The figure shows three views and two pictorial views of one solid part (mm, origin at its lowest corner). Answer the questions. A direction names the side the tool comes from. Coordinates: 2 decimals unless noted, no trailing zeros. Loops run counter-clockwise (first coordinate to the right, second up) from the corner with the lowest first, then second, coordinate; pieces in that order, holes last. Notation, with made-up numbers: M 65,-15 L 87,-15 A12 cw 87,-2 Z; hole C 70,-26 d5. An arc over 180 degrees is marked long. One line per item, written item: value. Start each with the question number.
1. Consider probe 1 along Y at (x, z) = (93.5, 25.5); probe 2 along Y at (x, z) = (13, 10.5); probe 3 along X at (y, z) = (47.5, 30). Determine where each line is inside the solid, lowest interval first.
2. For the marked faces 1, 2 and 3, determine the directions among +Z, -Z, +X, -X, +Y, -Y from which every point of the face is accessible in a straight line to the end or side of a thin tool.
3. Flat-ended cylindrical pins translate along their axes: pin 1 (16.5 mm diameter, centred on y = 45.5, z = 19.5, fed in from +X); pin 2 (6 mm diameter, centred on x = 78.5, z = 16, fed in from -Y); pin 3 (8 mm diameter, centred on y = 11, z = 49.5, fed in from -X) (3 decimals); pin 4 (3 mm diameter, centred on y = 31.5, z = 32.5, fed in from -X). Find the tip coordinate at first contact, or state that the pin passes through.
4. The part is cut by section A-A (y = 26.5). Write down the section's boundary in (x, z).
5. The part is cut by section B-B (x = 49.5). Write down the section's boundary in (y, z).
6. The part is cut by section C-C (y = 12.5). Write down the section's boundary in (x, z), then the cut area to 3 significant figures.
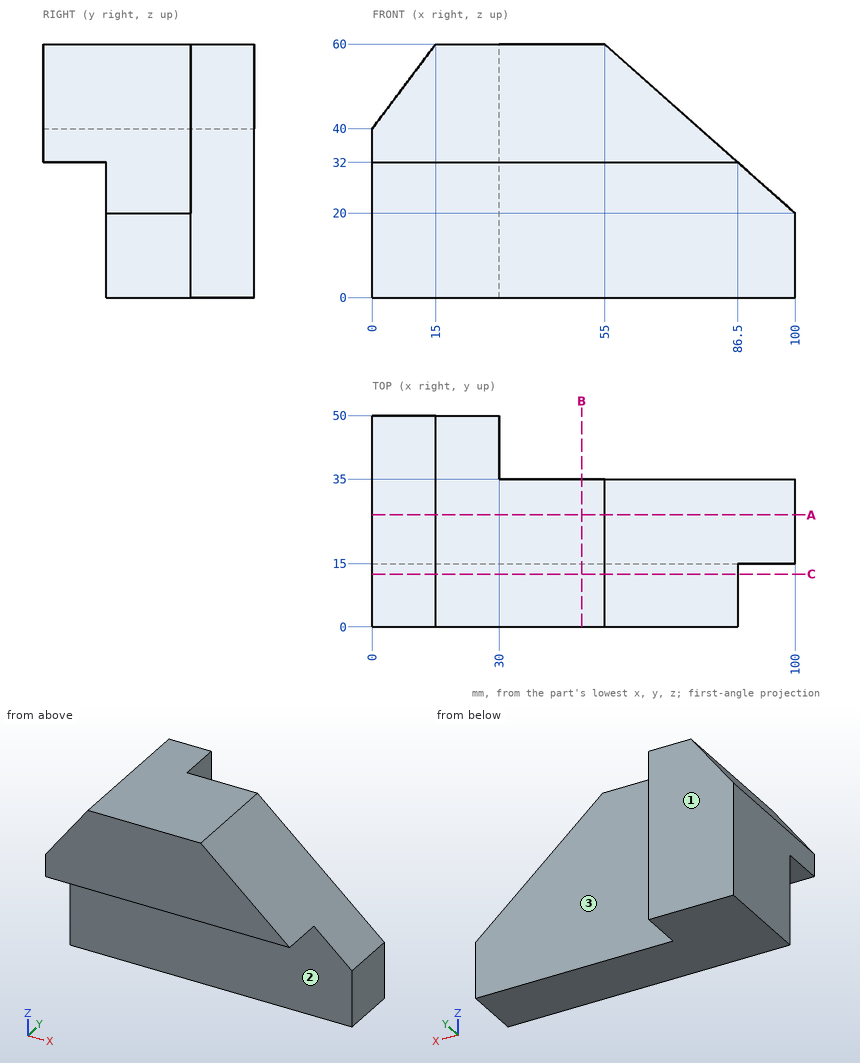
Answer block:
1. probe 1: y = 15 to 35
1. probe 2: y = 15 to 50
1. probe 3: x = 0 to 30
2. face 1: +Z, -Z, +X, -X, +Y
2. face 2: -Z, +X, -X, -Y
2. face 3: +Z, -Z, +X, +Y
3. pin 1: stops at x = 30
3. pin 2: stops at y = 15
3. pin 3: stops at x = 4.125
3. pin 4: stops at x = 0
4. outline: M 0,0 L 100,0 L 100,20 L 55,60 L 15,60 L 0,40 Z
5. outline: M 0,32 L 15,32 L 15,0 L 35,0 L 35,60 L 0,60 Z
6. outline: M 0,32 L 86.5,32 L 55,60 L 15,60 L 0,40 Z
6. area: 1,830 mm2
